For this review, use the dimensioned drawing (mm, ordinates from the lowest corner) and the shaded views. A direction names the side the tool comes from. Coordinates: 2 decimals unless noted, no trailing zeros. Loops run counter-clockwise (first coordinate to the right, second up) from the corner with the lowest first, then second, coordinate; pieces in that order, holes last. Notation, with made-up numbers: M 83.25,51.5 L 140.25,51.5 A35 ccw 140.25,84.5 Z; hole C -7,75.25 d1. An arc over 180 degrees is marked long. One line per item, written item: value.
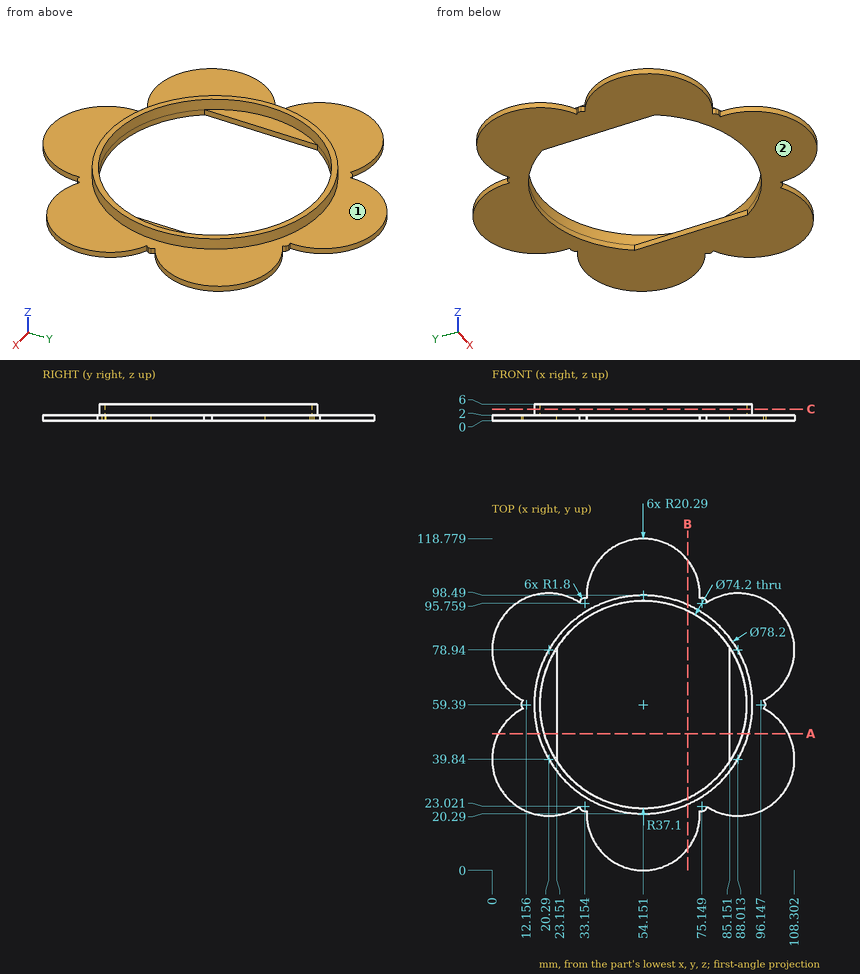
(1) We need section A-A on y = 49. State the section outline as (x, z) points (1 decimal).
Reply:
outline: M 2.2,0 L 23.2,0 L 23.2,2 L 18.5,2 L 18.5,6 L 16.5,6 L 16.5,2 L 2.2,2 Z; M 85.2,0 L 106.1,0 L 106.1,2 L 91.8,2 L 91.8,6 L 89.8,6 L 89.8,2 L 85.2,2 Z
(2) Tool access review of the marked faces 1 and 2: name each direction out of +Z, -Z, +X, -X, +Y, -Y from which nothing blocks a thin tool from reaching the whole face with its end or side.
Reply:
face 1: +Z
face 2: -Z, +X, -X, +Y, -Y
(3) We need section C-C on z = 4.15. State the section outline as (x, y) points.
Reply:
outline: C 54.15,59.39 d78.2; hole C 54.15,59.39 d74.2
(4) To check wall thickness, follow line 1 along Y through (x, z) = (55, 3); line 2 along Z through (x, y) = (35, 17.5); line 3 along X through (y, z) = (43.5, 5) (1 decimal). State the ranges of each line that lie inside material, in increasing order. Write a range as [from, to].
Reply:
line 1: y = [20.3, 22.3], [96.48, 98.48]
line 2: z = [0, 2]
line 3: x = [18.4, 20.6], [87.7, 89.9]
(5) Insertion check: pin 1 (1 mm diameter, centred on y = 25, z = 1, fed in from -X) (1 decimal); pin 2 (1 mm diameter, centred on y = 58.5, z = 1, fed in from +X); pin 3 (3 mm diameter, centred on x = 20, y = 69, fed in from +Z). Each pin has a flat end and moves straight along its axis. Give the tip position at first contact, or say it passes through.
Reply:
pin 1: stops at x = 5.9
pin 2: stops at x = 97.9
pin 3: stops at z = 2
(6) We need section B-B on x = 70. State the section outline as (y, z) points (1 decimal).
Reply:
outline: M 7.6,0 L 25.8,0 L 25.8,6 L 23.6,6 L 23.6,2 L 7.6,2 Z; M 92.9,0 L 111.2,0 L 111.2,2 L 95.1,2 L 95.1,6 L 92.9,6 Z
